```python
from build123d import *

# Parameters (mm, degrees)
F0_W     = 22.5
F0_H     = 65
F0_R     = 1.5
F1_DEPTH = 25
F3_DEPTH = 10


with BuildPart() as f1:
    # F0 (on Front) → F1 (new body)
    with BuildSketch(Plane.XZ):
        Rectangle(F0_W, F0_H)
        with Locations((-9.25, 0.5)):
            Circle(F0_R, mode=Mode.SUBTRACT)
        with Locations((9.25, 0.5)):
            Circle(F0_R, mode=Mode.SUBTRACT)
    extrude(amount=F1_DEPTH)

    # F2 (on face) → F3 (join)
    with BuildSketch(Plane.XZ.offset(25)):
        with BuildLine():
            Line((-2, 23.486068), (-2, 19.013932))
            ThreePointArc((-2, 19.013932), (0, 18.25), (2, 19.013932))
            Line((2, 19.013932), (2, 23.486068))
            ThreePointArc((2, 23.486068), (0, 24.25), (-2, 23.486068))
        make_face()
    extrude(amount=F3_DEPTH)


solid = f1.part
```
Geometry: final body of the model. Coordinates: model frame, mm. A direction names the side the tool comes from. Coordinates: 2 decimals unless noted, no trailing zeros. Loops run counter-clockwise (first coordinate to the right, second up) from the corner with the lowest first, then second, coordinate; pieces in that order, holes last. Notation, with made-up numbers: M -14.75,57.25 L -2.75,57.25 A20 ccw -2.75,95.25 Z; hole C 25.25,-8 d4. An arc over 180 degrees is marked long. Put each result on its own line as item: value.
(1) Cut plane B-B on x = 9.25. Return the cut outline in (y, z).
Answer sheet:
outline: M -25,-32.5 L 0,-32.5 L 0,-1 L -25,-1 Z; M -25,2 L 0,2 L 0,32.5 L -25,32.5 Z
(2) Cut plane A-A on z = 0.5. Return the cut outline in (x, y).
Answer sheet:
outline: M -11.25,-25 L -10.75,-25 L -10.75,0 L -11.25,0 Z; M -7.75,-25 L 7.75,-25 L 7.75,0 L -7.75,0 Z; M 10.75,-25 L 11.25,-25 L 11.25,0 L 10.75,0 Z
(3) Draft query along Z for faces 1 (the face through (0, -12, -32.5)), 2 (the face through (0.03, -29.93, 24.25)), 3 (the face through (-10.75, -12.32, 0.57)). Return one class per face: pulls with the +Z half, pulls with the -Z half, needs draft (parallel to the pull), parting line crosses it, or undercut.
Answer sheet:
face 1: pulls with the -Z half
face 2: pulls with the +Z half
face 3: undercut
(4) Access query for faces 4 (the face through (8.06, -12.32, -0.41)), 5 (the face through (-2, -30, 21)), 6 (the face through (2, -30, 21)), 7 (the face through (-0.03, -29.93, 18.25)), 8 (the face through (11.25, -12, 0)). Directions: +Z, -Z, +X, -X, +Y, -Y. A direction counts if a zero-diameter tool reaches every point of the face in a straight line with its end or side. Return the directions, or none.
Answer sheet:
face 4: +Y, -Y
face 5: +Z, -Z, -X, -Y
face 6: +Z, -Z, +X, -Y
face 7: -Z, -Y
face 8: +Z, -Z, +X, +Y, -Y
(5) Material intervals for probe 1 along X at (y, z) = (-16, 0); probe 2 along Z at (x, y) = (9.25, -11.5); probe 3 along Y at (x, z) = (-2.5, 22), sorted ascending.
Answer sheet:
probe 1: x = -11.25 to -10.66, -7.84 to 7.84, 10.66 to 11.25
probe 2: z = -32.5 to -1, 2 to 32.5
probe 3: y = -25 to 0
(6) Cut plane C-C on x = -3.5. Return the cut outline in (y, z).
Answer sheet:
outline: M -25,-32.5 L 0,-32.5 L 0,32.5 L -25,32.5 Z
(7) First-contact query: pin 1 (5 mm diameter, centred on x = -6, z = -12.5, fed in from -Y); pin 2 (2 mm diameter, centred on y = -28.5, z = 22, fed in from +X); pin 3 (1.5 mm diameter, centred on x = -3.5, y = -26, fed in from +Z); pin 4 (5 mm diameter, centred on y = -28, z = 22.5, fed in from -X). Flat tips, straight axial feed; report the tip coordinate or a pass-through.
Answer sheet:
pin 1: stops at y = -25
pin 2: stops at x = 2
pin 3: passes through
pin 4: stops at x = -2
(8) Cut plane D-D on z = 28. Return the cut outline in (x, y), then the cut area to 4 significant figures.
Answer sheet:
outline: M -11.25,-25 L 11.25,-25 L 11.25,0 L -11.25,0 Z
area: 562.5 mm^2
